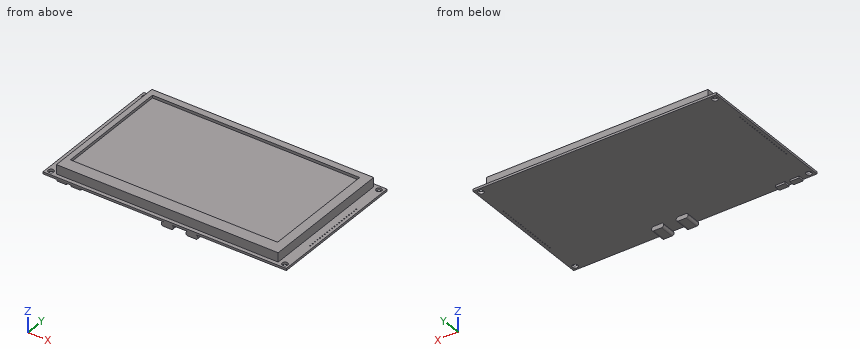
```python
from build123d import *

# Parameters (mm, degrees)
SKETCH1_W               = 180.9
SKETCH1_H               = 105.45
SKETCH1_R               = 2.05
BOSS_EXTRUDE1_DEPTH     = 0.8
SKETCH2_W               = 164.9
SKETCH2_H               = 100
BOSS_EXTRUDE2_DEPTH     = 6.83
BOSS_EXTRUDE3_DEPTH     = 11
SKETCH4_W               = 7
SKETCH4_H               = 4
BOSS_EXTRUDE4_DEPTH     = 1.5
CUT_EXTRUDE1_DEPTH      = 106.034246915
CUT_EXTRUDE1_DEPTH_BACK = 106.034246915
SKETCH5_R               = 0.38
SKETCH6_W               = 154.08
SKETCH6_H               = 85.92
CUT_EXTRUDE2_DEPTH      = 2


with BuildPart() as part:
    # Sketch1 → Boss-Extrude1 (new, symmetric)
    with BuildSketch(Plane.XY):
        Rectangle(SKETCH1_W, SKETCH1_H)
        with Locations((86.95, 49.245)):
            Circle(SKETCH1_R, mode=Mode.SUBTRACT)
        with Locations((-86.96, 49.245)):
            Circle(SKETCH1_R, mode=Mode.SUBTRACT)
        with Locations((-86.96, -49.225)):
            Circle(SKETCH1_R, mode=Mode.SUBTRACT)
        with Locations((86.95, -49.225)):
            Circle(SKETCH1_R, mode=Mode.SUBTRACT)
    extrude(amount=BOSS_EXTRUDE1_DEPTH, both=True)

    # Sketch2 → Boss-Extrude2 (add)
    with BuildSketch(Plane.XY.offset(0.8)):
        with Locations((0, 0.045)):
            Rectangle(SKETCH2_W, SKETCH2_H)
    extrude(amount=BOSS_EXTRUDE2_DEPTH)

    # Sketch3 → Boss-Extrude3 (add)
    with BuildSketch(Plane.XZ.offset(52.725)):
        with BuildLine():
            Line((17.37, -0.8), (23.15, -0.8))
            ThreePointArc((23.15, -0.8), (24.267228714, -1.262771286), (24.73, -2.38))
            Line((24.73, -2.38), (24.73, -2.48))
            ThreePointArc((24.73, -2.48), (24.267228714, -3.597228714), (23.15, -4.06))
            Line((23.15, -4.06), (17.37, -4.06))
            ThreePointArc((17.37, -4.06), (16.252771286, -3.597228714), (15.79, -2.48))
            Line((15.79, -2.48), (15.79, -2.38))
            ThreePointArc((15.79, -2.38), (16.252771286, -1.262771286), (17.37, -0.8))
        make_face()
        with BuildLine():
            Line((-0.91, -0.8), (4.87, -0.8))
            ThreePointArc((4.87, -0.8), (5.987228714, -1.262771286), (6.45, -2.38))
            Line((6.45, -2.38), (6.45, -2.48))
            ThreePointArc((6.45, -2.48), (5.987228714, -3.597228714), (4.87, -4.06))
            Line((4.87, -4.06), (-0.91, -4.06))
            ThreePointArc((-0.91, -4.06), (-2.027228714, -3.597228714), (-2.49, -2.48))
            Line((-2.49, -2.48), (-2.49, -2.38))
            ThreePointArc((-2.49, -2.38), (-2.027228714, -1.262771286), (-0.91, -0.8))
        make_face()
    extrude(amount=-BOSS_EXTRUDE3_DEPTH)

    # Sketch4 → Boss-Extrude4 (add)
    with BuildSketch(Plane(origin=(0, 0, -0.8), x_dir=(-1, 0, 0), z_dir=(0, 0, -1))):
        with Locations((66.42, -50.205)):
            Rectangle(SKETCH4_W, SKETCH4_H)
        with Locations((76.91, -50.205)):
            Rectangle(SKETCH4_W, SKETCH4_H)
    extrude(amount=BOSS_EXTRUDE4_DEPTH)

    # Sketch5 → Cut-Extrude1 (cut, two sides: drawn at the far end of the back side and taken through both)
    with BuildSketch(Plane(origin=(0, 0, -0.8), x_dir=(-1, 0, 0), z_dir=(0, 0, -1)).offset(-CUT_EXTRUDE1_DEPTH_BACK)):
        with Locations(Location((87.95, 24.125, 0), (0, 0, 180))):
            Circle(SKETCH5_R)
        with Locations(Location((87.95, 21.585, 0), (0, 0, 180))):
            Circle(SKETCH5_R)
        with Locations(Location((87.95, 19.045, 0), (0, 0, 180))):
            Circle(SKETCH5_R)
        with Locations(Location((87.95, 16.505, 0), (0, 0, 180))):
            Circle(SKETCH5_R)
        with Locations(Location((87.95, 13.965, 0), (0, 0, 180))):
            Circle(SKETCH5_R)
        with Locations(Location((87.95, 11.425, 0), (0, 0, 180))):
            Circle(SKETCH5_R)
        with Locations(Location((87.95, 8.885, 0), (0, 0, 180))):
            Circle(SKETCH5_R)
        with Locations(Location((87.95, 6.345, 0), (0, 0, 180))):
            Circle(SKETCH5_R)
        with Locations(Location((87.95, 3.805, 0), (0, 0, 180))):
            Circle(SKETCH5_R)
        with Locations(Location((87.95, 1.265, 0), (0, 0, 180))):
            Circle(SKETCH5_R)
        with Locations(Location((87.95, -1.275, 0), (0, 0, 180))):
            Circle(SKETCH5_R)
        with Locations(Location((87.95, -3.815, 0), (0, 0, 180))):
            Circle(SKETCH5_R)
        with Locations(Location((87.95, -6.355, 0), (0, 0, 180))):
            Circle(SKETCH5_R)
        with Locations(Location((87.95, -8.895, 0), (0, 0, 180))):
            Circle(SKETCH5_R)
        with Locations(Location((87.95, -11.435, 0), (0, 0, 180))):
            Circle(SKETCH5_R)
        with Locations(Location((87.95, -13.975, 0), (0, 0, 180))):
            Circle(SKETCH5_R)
        with Locations(Location((87.95, -16.515, 0), (0, 0, 180))):
            Circle(SKETCH5_R)
        with Locations(Location((87.95, -19.055, 0), (0, 0, 180))):
            Circle(SKETCH5_R)
        with Locations(Location((87.95, -21.595, 0), (0, 0, 180))):
            Circle(SKETCH5_R)
        with Locations(Location((87.95, -24.135, 0), (0, 0, 180))):
            Circle(SKETCH5_R)
        with Locations(Location((-87.96, 24.095, 0), (0, 0, 180))):
            Circle(SKETCH5_R)
        with Locations(Location((-87.96, 21.555, 0), (0, 0, 180))):
            Circle(SKETCH5_R)
        with Locations(Location((-87.96, 19.015, 0), (0, 0, 180))):
            Circle(SKETCH5_R)
        with Locations(Location((-87.96, 16.475, 0), (0, 0, 180))):
            Circle(SKETCH5_R)
        with Locations(Location((-87.96, 13.935, 0), (0, 0, 180))):
            Circle(SKETCH5_R)
        with Locations(Location((-87.96, 11.395, 0), (0, 0, 180))):
            Circle(SKETCH5_R)
        with Locations(Location((-87.96, 8.855, 0), (0, 0, 180))):
            Circle(SKETCH5_R)
        with Locations(Location((-87.96, 6.315, 0), (0, 0, 180))):
            Circle(SKETCH5_R)
        with Locations(Location((-87.96, 3.775, 0), (0, 0, 180))):
            Circle(SKETCH5_R)
        with Locations(Location((-87.96, 1.235, 0), (0, 0, 180))):
            Circle(SKETCH5_R)
        with Locations(Location((-87.96, -1.305, 0), (0, 0, 180))):
            Circle(SKETCH5_R)
        with Locations(Location((-87.96, -3.845, 0), (0, 0, 180))):
            Circle(SKETCH5_R)
        with Locations(Location((-87.96, -6.385, 0), (0, 0, 180))):
            Circle(SKETCH5_R)
        with Locations(Location((-87.96, -8.925, 0), (0, 0, 180))):
            Circle(SKETCH5_R)
        with Locations(Location((-87.96, -11.465, 0), (0, 0, 180))):
            Circle(SKETCH5_R)
        with Locations(Location((-87.96, -14.005, 0), (0, 0, 180))):
            Circle(SKETCH5_R)
        with Locations(Location((-87.96, -16.545, 0), (0, 0, 180))):
            Circle(SKETCH5_R)
        with Locations(Location((-87.96, -19.085, 0), (0, 0, 180))):
            Circle(SKETCH5_R)
        with Locations(Location((-87.96, -21.625, 0), (0, 0, 180))):
            Circle(SKETCH5_R)
        with Locations(Location((-87.96, -24.165, 0), (0, 0, 180))):
            Circle(SKETCH5_R)
    extrude(amount=CUT_EXTRUDE1_DEPTH + CUT_EXTRUDE1_DEPTH_BACK, mode=Mode.SUBTRACT)

    # Sketch6 → Cut-Extrude2 (cut)
    with BuildSketch(Plane.XY.offset(7.63)):
        with Locations((-1.48, 2.085)):
            Rectangle(SKETCH6_W, SKETCH6_H)
    extrude(amount=-CUT_EXTRUDE2_DEPTH, mode=Mode.SUBTRACT)


solid = part.part
```
Can you work these out from the model? Positions are in its coordinate system, mm. Give positions to 0.01 mm unless a question says otherwise; leave off trailing zeros. Order: outer loops, then holes, each group sorted by start corner. A loop starts at its lowest first (then second) coordinate and runs counter-clockwise, first axis right, second up. Notation, with made-up numbers: (2.5, -12) - (10.5, -12) arc R20 cw to (10.5, -3) - close; hole circle Ø8 at (20, -23.75). An arc over 180 degrees is marked (long way). Use a Markdown table: item, result. Add a question column.
Q1. I'm going to push flat-ended pins straight in: pin 1 (3 mm diameter, centred on x = -76.5, y = -50, fed in from -Z); pin 2 (4 mm diameter, centred on x = 57, y = -41, fed in from -Z); pin 3 (1.2 mm diameter, centred on y = -51, z = -1.5, fed in from +X) (3 decimals). Where does each tip first touch, or does it pass through?
Q2. If we section it at D-D on z = 3: Write out the boundary of the cut face in (x, y) (3 decimals).
Q3. If we section it at B-B on x = -68: Write out the boundary of the cut face in (y, z) (3 decimals).
Q4. If we section it at C-C on y = -45: Write out the boundary of the cut face in (x, z).
Q5. Please list where these lines run through material, in increasing order: line 1 along Y through (x, z) = (-86.96, -0.15) (3 decimals); line 2 along X through (y, z) = (33.5, 6); line 3 along X through (y, z) = (16.5, -0.75).
Q6. If we section it at A-A on y = -32: Write out the boundary of the cut face in (x, z), plus the area to 3 significant figures.
Answers follow:
| question | item | result |
|---|---|---|
| 1 | pin 1 | stops at z = -2.3 |
| 1 | pin 2 | stops at z = -0.8 |
| 1 | pin 3 | stops at x = 24.705 |
| 2 | outline | (-82.45, -49.955) - (82.45, -49.955) - (82.45, 50.045) - (-82.45, 50.045) - close |
| 3 | outline | (-52.725, -0.8) - (-52.205, -0.8) - (-52.205, -2.3) - (-48.205, -2.3) - (-48.205, -0.8) - (52.725, -0.8) - (52.725, 0.8) - (50.045, 0.8) - (50.045, 7.63) - (45.045, 7.63) - (45.045, 5.63) - (-40.875, 5.63) - (-40.875, 7.63) - (-49.955, 7.63) - (-49.955, 0.8) - (-52.725, 0.8) - close |
| 4 | outline | (-90.45, -0.8) - (-0.91, -0.8) arc R1.58 ccw to (-2.49, -2.38) - (-2.49, -2.48) arc R1.58 ccw to (-0.91, -4.06) - (4.87, -4.06) arc R1.58 ccw to (6.45, -2.48) - (6.45, -2.38) arc R1.58 ccw to (4.87, -0.8) - (17.37, -0.8) arc R1.58 ccw to (15.79, -2.38) - (15.79, -2.48) arc R1.58 ccw to (17.37, -4.06) - (23.15, -4.06) arc R1.58 ccw to (24.73, -2.48) - (24.73, -2.38) arc R1.58 ccw to (23.15, -0.8) - (90.45, -0.8) - (90.45, 0.8) - (82.45, 0.8) - (82.45, 7.63) - (-82.45, 7.63) - (-82.45, 0.8) - (-90.45, 0.8) - close |
| 5 | line 1 | y = -52.725 to -51.275, -47.175 to 47.195, 51.295 to 52.725 |
| 5 | line 2 | x = -82.45 to -78.52, 75.56 to 82.45 |
| 5 | line 3 | x = -90.45 to -88.33, -87.57 to 87.58, 88.34 to 90.45 |
| 6 | outline | (-90.45, -0.8) - (90.45, -0.8) - (90.45, 0.8) - (82.45, 0.8) - (82.45, 7.63) - (75.56, 7.63) - (75.56, 5.63) - (-78.52, 5.63) - (-78.52, 7.63) - (-82.45, 7.63) - (-82.45, 0.8) - (-90.45, 0.8) - close |
| 6 | area | 1,110 mm^2 |
